For this review, take the finished solid that the model builds, in its own axes (mm). A direction names the side the tool comes from. Coordinates: 2 decimals unless noted, no trailing zeros. Loops run counter-clockwise (first coordinate to the right, second up) from the corner with the lowest first, then second, coordinate; pieces in that order, holes last. Notation, with made-up numbers: (-1.5, -10.75) - (12.5, -10.75) arc R30 ccw to (12.5, 16.25) - close; hole circle Ø3 at (-31.75, 5). An arc over 180 degrees is marked (long way). One line per item, written item: value. Start each with the question number.
1. Take a section at D-D, the plane x = 182. State the section outline as (y, z) points, and give its area (3 significant figures).
2. For faces 1 (the face through (-469, -150, 338)), 2 (the face through (-101.217, -223.95, 166.051)), 3 (the face through (-500, -2, 173)), 4 (the face through (-7, 2, 0)), list the 3-axis set-ups (+Z, -Z, +X, -X, +Y, -Y) from which the entire face can be reached by the end or side of a thin tool; tool diameter is ignored.
3. Take a section at C-C, the plane y = -80.5. State the section outline as (x, z) points, and give its area (3 significant figures).
4. Take a section at A-A, the plane x = -282. State the section outline as (y, z) points.
5. To check wall thickness, follow line 1 (X direction, y = 121, z = 37); line 2 (Y direction, x = 363.5, z = 161); line 3 (Z direction, x = -257, y = 73). State the ranges of each line that lie inside material, in increasing order. Write a range as from..to.
6. Insertion check: pin 1 (1 mm diameter, centred on x = 88, y = 25, fed in from -Z); pin 2 (3 mm diameter, centred on x = 43.5, z = 2.5, fed in from -Y); pin 3 (3 mm diameter, centred on x = -84.5, y = 24.5, fed in from +Z). Each pin has a flat end and moves straight along its axis. Give the tip position at first contact, or say it passes through.
7. Take a section at B-B, the plane z = 175.5. State the section outline as (x, y) points, and give its area (3 significant figures).
```python
from build123d import *

# Parameters (mm, degrees)
F0_W     = 1000
F0_H     = 300
F1_DEPTH = 350
F2_R     = 265.5
F2_R_2   = 190.5
F3_DEPTH = 150


with BuildPart() as f1:
    # F0 (on Top) → F1 (new body)
    with BuildSketch(Plane.XY):
        Rectangle(F0_W, F0_H)
    extrude(amount=F1_DEPTH)

    # F2 (on face) → F3 (join)
    with BuildSketch(Plane.XZ.offset(150)):
        with Locations((-354.456395, 86.301595)):
            Circle(F2_R)
        with Locations((-354.456395, 86.301595)):
            Circle(F2_R_2, mode=Mode.SUBTRACT)
        with BuildLine():
            Line((-500, 0), (-500, 209.213389))
            ThreePointArc((-500, 209.213389), (-459.765558, -72.444209), (-184.626231, 0))
            Line((-184.626231, 0), (-500, 0))
        make_face()
        with BuildLine():
            ThreePointArc((-184.626231, 0), (-169.195908, 41.930412), (-163.956395, 86.301595))
            ThreePointArc((-163.956395, 86.301595), (-289.018664, 265.209821), (-500, 209.213389))
            Line((-500, 209.213389), (-500, 0))
            Line((-500, 0), (-184.626231, 0))
        make_face()
    extrude(amount=F3_DEPTH)


solid = f1.part
```
Solutions:
1. outline: (-150, 0) - (150, 0) - (150, 350) - (-150, 350) - close
1. area: 105,000 mm2
2. face 1: +Z, -X, -Y
2. face 2: -Y
2. face 3: +Z, -Z, -X, +Y
2. face 4: -Z, +X, -X, +Y
3. outline: (-500, 0) - (500, 0) - (500, 350) - (-500, 350) - close
3. area: 350,000 mm2
4. outline: (-300, -169.12) - (-150, -169.12) - (-150, 0) - (150, 0) - (150, 350) - (-150, 350) - (-150, 341.72) - (-300, 341.72) - close
5. line 1: -500..500
5. line 2: -150..150
5. line 3: 0..350
6. pin 1: z = 0
6. pin 2: y = -150
6. pin 3: z = 350
7. outline: (-604.52, -300) - (-104.39, -300) - (-104.39, -150) - (500, -150) - (500, 150) - (-500, 150) - (-500, -150) - (-604.52, -150) - close
7. area: 375,000 mm2
